Check sheet for the modelled part. Datum: model origin and axes. Units: mm. Round coordinates to 2 decimals unless told otherwise and drop trailing zeros. Return JSON: item names as keys, results as strings.
Autodesk Inventor part; units mm, degrees
ref_plane "Work Plane4" through (0, 0, 0) normal (0, 1, 0) x (-1, 0, 0)
ref_plane "Work Plane5" through (0, -10, 0) normal (0, 1, 0) x (-1, 0, 0)
ref_plane "YZ Plane" through (0, 0, 0) normal (1, 0, 0) x (0, 1, 0)
sketch "Sketch1" plane through (0, 0, 0) normal (0, 0, 1) x (1, 0, 0)
  line L0 (-3.9007, 3.9007) -> (3.9007, 3.9007)
  line L1 (3.9007, 3.9007) -> (3.9007, -3.9007)
  line L2 (3.9007, -3.9007) -> (-3.9007, -3.9007)
  line L3 (-3.9007, -3.9007) -> (-3.9007, 3.9007)
  line L4 (0, 3.9007) -> (0, -3.9007) construction
  line L5 (-3.9007, 0) -> (3.9007, 0) construction
  circle A0 centre (0, 0) radius 2.1
  line L6 (0, 0) -> (-16.1173, 16.1173) construction
  line L7 (0, 0) -> (22.7933, 0) construction
  line L8 (-2.84, 3.9007) -> (-5.4993, 6.56)
  line L9 (-5.4993, 6.56) -> (-5.4993, 8.2)
  line L10 (-5.4993, 8.2) -> (-2.84, 8.2)
  line L11 (-2.84, 8.2) -> (-4.64, 10)
  line L12 (-4.64, 10) -> (-10, 10)
  line L13 (-10, 10) -> (-10, 4.64)
  line L14 (-10, 4.64) -> (-8.2, 2.84)
  line L15 (-8.2, 2.84) -> (-8.2, 5.4993)
  line L16 (-8.2, 5.4993) -> (-6.56, 5.4993)
  line L17 (-6.56, 5.4993) -> (-3.9007, 2.84)
  line L18 (-3.9007, 2.84) -> (-11.3102, 2.84) construction
  line L19 (-2.84, 3.9007) -> (-3.9007, 3.9007)
  line L20 (-3.9007, 2.84) -> (-3.9007, 3.9007)
  line L21 (-3.9007, -2.84) -> (-6.56, -5.4993)
  line L22 (-6.56, -5.4993) -> (-8.2, -5.4993)
  line L23 (-8.2, -5.4993) -> (-8.2, -2.84)
  line L24 (-8.2, -2.84) -> (-10, -4.64)
  line L25 (-10, -4.64) -> (-10, -10)
  line L26 (-10, -10) -> (-4.64, -10)
  line L27 (-4.64, -10) -> (-2.84, -8.2)
  line L28 (-2.84, -8.2) -> (-5.4993, -8.2)
  line L29 (-5.4993, -8.2) -> (-5.4993, -6.56)
  line L30 (-5.4993, -6.56) -> (-2.84, -3.9007)
  line L31 (-3.9007, -2.84) -> (-3.9007, -3.9007)
  line L32 (-2.84, -3.9007) -> (-3.9007, -3.9007)
  line L33 (2.84, -3.9007) -> (5.4993, -6.56)
  line L34 (5.4993, -6.56) -> (5.4993, -8.2)
  line L35 (5.4993, -8.2) -> (2.84, -8.2)
  line L36 (2.84, -8.2) -> (4.64, -10)
  line L37 (4.64, -10) -> (10, -10)
  line L38 (10, -10) -> (10, -4.64)
  line L39 (10, -4.64) -> (8.2, -2.84)
  line L40 (8.2, -2.84) -> (8.2, -5.4993)
  line L41 (8.2, -5.4993) -> (6.56, -5.4993)
  line L42 (6.56, -5.4993) -> (3.9007, -2.84)
  line L43 (2.84, -3.9007) -> (3.9007, -3.9007)
  line L44 (3.9007, -2.84) -> (3.9007, -3.9007)
  line L45 (3.9007, 2.84) -> (6.56, 5.4993)
  line L46 (6.56, 5.4993) -> (8.2, 5.4993)
  line L47 (8.2, 5.4993) -> (8.2, 2.84)
  line L48 (8.2, 2.84) -> (10, 4.64)
  line L49 (10, 4.64) -> (10, 10)
  line L50 (10, 10) -> (4.64, 10)
  line L51 (4.64, 10) -> (2.84, 8.2)
  line L52 (2.84, 8.2) -> (5.4993, 8.2)
  line L53 (5.4993, 8.2) -> (5.4993, 6.56)
  line L54 (5.4993, 6.56) -> (2.84, 3.9007)
  line L55 (3.9007, 2.84) -> (3.9007, 3.9007)
  line L56 (2.84, 3.9007) -> (3.9007, 3.9007)
  dimension "d7" = 4.2
  dimension "d8" = 135
  dimension "d9" = 1.5
  dimension "d10" = 1.64
  dimension "d11" = 1.8
  dimension "d12" = 2.84
  dimension "d13" = 10
  dimension "d16" = 360
extrude "Extrusion1" add sketch "Sketch1" along normal blind 700
pattern_linear "Rectangular Pattern1" count 2 spacing 20 along (0, -1, 0) of "Extrusion1"
sketch "Sketch2" plane through (0, 0, 700) normal (0, 0, 1) x (1, 0, 0)
  line L0 (8.2, -2.84) -> (8.2, -5.4993)
  line L1 (8.2, -5.4993) -> (6.56, -5.4993)
  line L2 (-6.56, -5.4993) -> (-8.2, -5.4993)
  line L3 (-8.2, -5.4993) -> (-8.2, -2.84)
  line L4 (-8.2, -14.5007) -> (-6.56, -14.5007)
  line L5 (6.56, -14.5007) -> (8.2, -14.5007)
  line L6 (5.4993, -11.8) -> (5.4993, -13.44)
  line L7 (5.4993, -13.44) -> (2.84, -16.0993)
  line L8 (-2.84, -16.0993) -> (-5.4993, -13.44)
  line L9 (-5.4993, -8.2) -> (-5.4993, -6.56)
  line L10 (-5.4993, -6.56) -> (-2.84, -3.9007)
  line L11 (2.84, -3.9007) -> (5.4993, -6.56)
  line L12 (2.84, -8.2) -> (4.64, -10)
  line L13 (-8.2, -6.9993) -> (-5.9387, -6.9993)
  line L14 (-5.9387, -6.9993) -> (-4.1231, -5.1837)
  line L15 (-4.1231, -5.1837) -> (4.1231, -5.1837)
  line L16 (4.1231, -5.1837) -> (5.9387, -6.9993)
  line L17 (5.9387, -6.9993) -> (8.2, -6.9993)
  line L18 (8.2, -6.9993) -> (8.2, -13.0007)
  line L19 (8.2, -13.0007) -> (5.9387, -13.0007)
  line L20 (5.9387, -13.0007) -> (4.2461, -14.6932)
  line L21 (4.2461, -14.6932) -> (-4.2461, -14.6932)
  line L22 (-4.2461, -14.6932) -> (-5.9387, -13.0007)
  line L23 (-5.9387, -13.0007) -> (-8.2, -13.0007)
  line L24 (-8.2, -13.0007) -> (-8.2, -6.9993)
  dimension "d23" = 1.5
  dimension "d24" = 1.5
  dimension "d25" = 1.5
  dimension "d26" = 1.5
extrude "Extrusion2" cut sketch "Sketch2" against normal up to next
ref_plane "Work Plane3" through (0, -20, 0) normal (0, 1, 0) x (-1, 0, 0)
ref_plane "Work Plane2" through (0, 0, 0) normal (0, 1, 0) x (-1, 0, 0)
ref_plane "Work Plane4" through (0, 0, 0) normal (0, 1, 0) x (-1, 0, 0)
ref_plane "Work Plane5" through (0, -10, 0) normal (0, 1, 0) x (-1, 0, 0)
ref_plane "Work Plane1" through (0, -10, 0) normal (0, 1, 0) x (-1, 0, 0)
equation "\"d24\" = d23"
equation "\"d25\" = d23"
equation "\"d26\" = d23"
properties part number "20x40x597mm" material "Aluminum 6061"
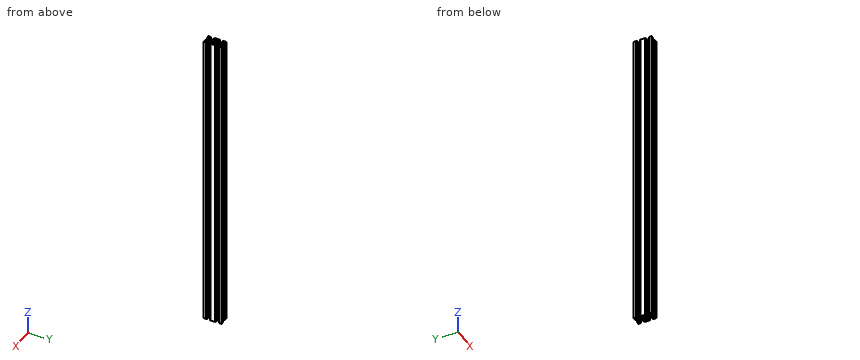
Q1. Section check A-A (z = 303.5). Count the separate pieces of the cut face and the enclosed holes in it, then the cut area to 3 significant figures.
Results list:
{"separate pieces": "1", "enclosed holes": "3", "area": "297 mm^2"}
Q2. Material ranges on line 1 (Y direction, x = 0, z = 311); line 2 (X direction, y = -0.5, z = 211.5); line 3 (Y direction, x = -4, z = 633), recorded low to high.
Results list:
{"line 1": "-23.9 to -22.1, -17.9 to -16.1, -3.9 to -2.1, 2.1 to 3.9", "line 2": "-3.9 to -2.04, 2.04 to 3.9", "line 3": "-29.36 to -28.2, -25.06 to -22.94, -17.06 to -14.94, -5.06 to -2.94, 2.94 to 5.06, 8.2 to 9.36"}
Q3. Go/stop test with flat-tipped pins: pin 1 (2 mm diameter, centred on x = 2.5, y = -19.5, fed in from -Z); pin 2 (0.8 mm diameter, centred on y = -23.5, z = 430.5, fed in from +X); pin 3 (4.5 mm diameter, centred on y = 0.5, z = 363.5, fed in from -X); pin 4 (3 mm diameter, centred on x = -0.5, z = 245.5, fed in from -Y). Record where each tip stops, or that it passes through.
Results list:
{"pin 1": "z = 0", "pin 2": "x = 9.26", "pin 3": "x = -3.9", "pin 4": "y = -23.9"}
